The figure shows three views and two pictorial views of one solid part (mm, origin at its lowest corner). Answer the questions. Round coordinates to 2 decimals unless told otherwise and drop trailing zeros. Write each loop counter-clockwise with the first axis right and the second up, starting at its lowest first coordinate (ties: lowest second). Pieces come first, ordered by that corner, then holes. Notation, with made-up numbers: M 21,42 L 61,42 A26 ccw 61,75 Z; hole C 1,-31 d3. An arc over 180 degrees is marked long. Use one line per item in the form item = value. Start each with the question number.
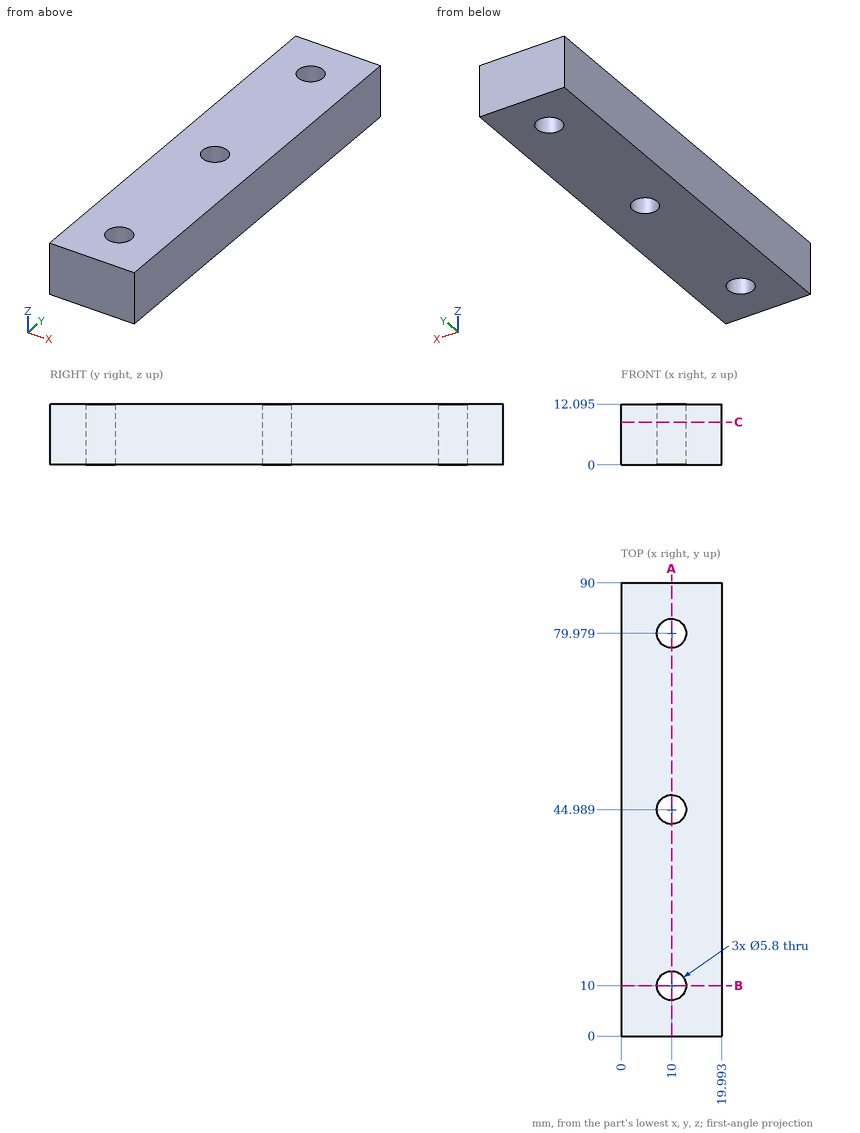
Q1. Straight lines are drawn through the part: line 1 (Y direction, x = 9.75, z = 4.75); line 2 (Y direction, x = 9.5, z = 9.5) (1 decimal); line 3 (X direction, y = 10, z = 4). For each, find the intervals that lie inside material, in ascending order. Write a range as [from, to].
Q2. Find section C-C on z = 8.5. Write down the section's boundary in (x, y).
Q3. Find section B-B on y = 10. Write down the section's boundary in (x, z) (1 decimal).
Q4. This flat-tipped pin is pushed along its axis until it touches: pin 1 Ø3 at (y, z) = (73, 3) entering from -X. Where does it stop, or does it pass through?
Q5. Find section A-A on x = 10. Write down the section's boundary in (y, z) (1 decimal).
Response:
q1.line_1 = [0, 7.11], [12.89, 42.1], [47.88, 77.09], [82.87, 90]
q1.line_2 = [0, 7.1], [12.9, 42.1], [47.8, 77.1], [82.8, 90]
q1.line_3 = [0, 7.1], [12.9, 19.99]
q2.outline = M 0,0 L 19.99,0 L 19.99,90 L 0,90 Z; hole C 10,10 d5.8; hole C 10,44.99 d5.8; hole C 10,79.98 d5.8
q3.outline = M 0,0 L 7.1,0 L 7.1,12.1 L 0,12.1 Z; M 12.9,0 L 20,0 L 20,12.1 L 12.9,12.1 Z
q4.pin_1 = 0
q5.outline = M 0,0 L 7.1,0 L 7.1,12.1 L 0,12.1 Z; M 12.9,0 L 42.1,0 L 42.1,12.1 L 12.9,12.1 Z; M 47.9,0 L 77.1,0 L 77.1,12.1 L 47.9,12.1 Z; M 82.9,0 L 90,0 L 90,12.1 L 82.9,12.1 Z
